Geometry check sheet. Reference: drawing and pictorial views, mm from the part's lowest x, y, z. A direction names the side the tool comes from. Give positions to 0.01 mm unless a question says otherwise; leave off trailing zeros. Write each loop counter-clockwise with the first axis right and the second up, starting at its lowest first coordinate (ties: lowest second). Pieces come first, ordered by that corner, then holes. Notation, with made-up numbers: (-31.75, 36.25) - (1.25, 36.25) arc R23 ccw to (1.25, 55.25) - close; hole circle Ø9 at (46.5, 6). An arc over 180 degrees is marked (long way). Write item = value, one per line. Start each with the question number.
(1) Section check A-A, the plane z = 15. Enter the section's corners in (x, y), plus the area to 3 significant figures.
(2) Thickness scan on L1, parallel to X at y = 425, z = 11.5; L2, parallel to Z at x = 181.5, y = 284; L3, parallel to X at y = 400, z = 23.5. Record the ranges inside material, lowest first.
(3) Section check D-D, the plane y = 77.5. Enter the section's corners in (x, z), plus the area to 4 significant figures.
(4) Depth check by flat-ended pin: pin 1 Ø24 at (x, y) = (222.5, 332.5) entering from +Z; pin 2 Ø3 at (y, z) = (321, 26) entering from +X; pin 3 Ø6 at (x, z) = (119.5, 26) entering from -Y; pin 4 Ø12 at (x, z) = (231, 22) entering from +Y. Enter the tip coordinate at first touch or a pass-through.
(5) Section check C-C, the plane x = 90. Enter the section's corners in (y, z), plus the area to 3 significant figures.
(6) Access from +Z, -Z, +X, -X, +Y, -Y to the whole of each face (thin tool, end or side, straight path). Record for the marked faces 1 and 2.
(7) Section check B-B, the plane y = 326. Enter the section's corners in (x, z).
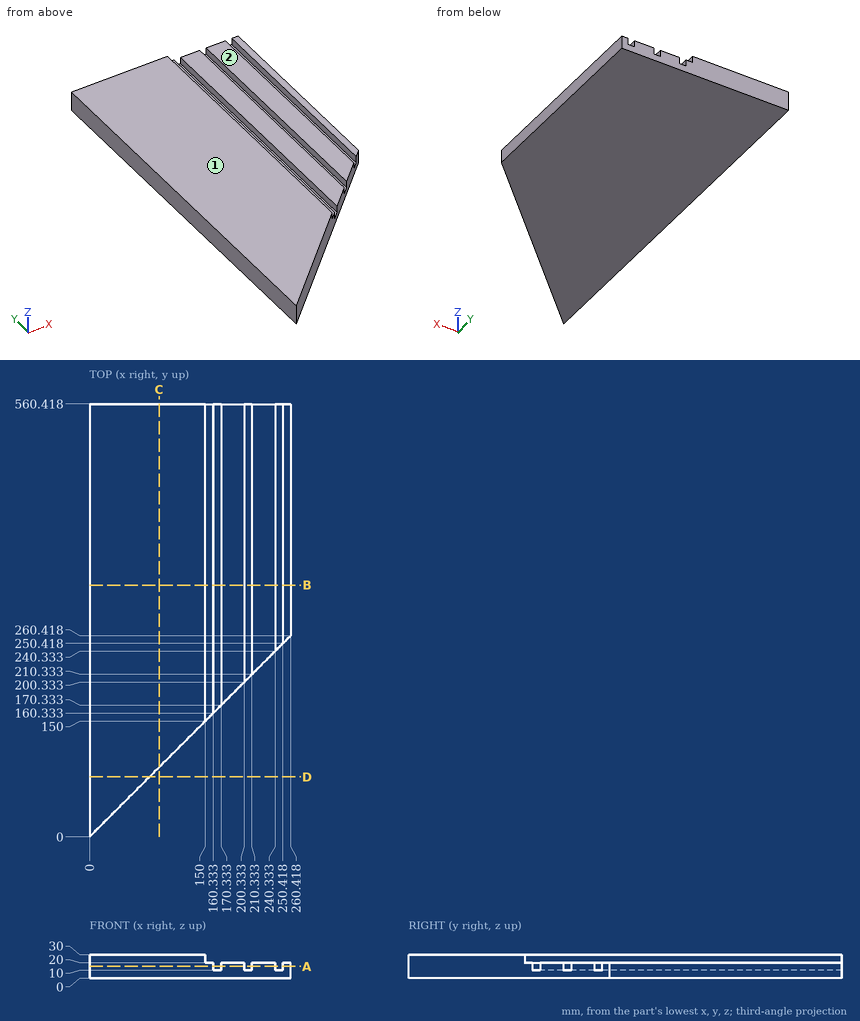
Model answer:
q1.outline = (0, 0) - (160.33, 160.33) - (160.33, 560.42) - (0, 560.42) - close; (170.33, 170.33) - (200.33, 200.33) - (200.33, 560.42) - (170.33, 560.42) - close; (210.33, 210.33) - (240.33, 240.33) - (240.33, 560.42) - (210.33, 560.42) - close; (250.42, 250.42) - (260.42, 260.42) - (260.42, 560.42) - (250.42, 560.42) - close
q1.area = 101,000 mm²
q2.L1 = 0 to 160.33, 170.33 to 200.33, 210.33 to 240.33, 250.42 to 260.42
q2.L2 = 0 to 20
q2.L3 = 0 to 150
q3.outline = (0, 0) - (77.5, 0) - (77.5, 30) - (0, 30) - close
q3.area = 2,325 mm²
q4.pin_1 = 20
q4.pin_2 = 150
q4.pin_3 = 116.5
q4.pin_4 = 560.42
q5.outline = (90, 0) - (560.42, 0) - (560.42, 30) - (90, 30) - close
q5.area = 14,100 mm²
q6.face_1 = +Z, +X, -X, +Y, -Y
q6.face_2 = +Z, +X, +Y, -Y
q7.outline = (0, 0) - (260.42, 0) - (260.42, 20) - (250.42, 20) - (250.42, 10) - (240.33, 10) - (240.33, 20) - (210.33, 20) - (210.33, 10) - (200.33, 10) - (200.33, 20) - (170.33, 20) - (170.33, 10) - (160.33, 10) - (160.33, 20) - (150, 20) - (150, 30) - (0, 30) - close
